Could you check a few things on this model? Use its own coordinates, in mm. A direction names the side the tool comes from. Round coordinates to 2 decimals unless told otherwise and drop trailing zeros. Write each loop counter-clockwise with the first axis right and the second up, starting at its lowest first coordinate (ties: lowest second). Pieces come first, ordered by that corner, then holes. Notation, with made-up numbers: (83.25, 73) -> (139.25, 73) arc R18 ccw to (139.25, 88) -> close; hole circle Ø6 at (36, 60.5). An arc over 180 degrees is marked (long way). Answer as CSV lines item,"result". Start each with the question number.
Q1. Imagine slicing it at C-C on y = 20. Please give me the cut outline in (x, z), and give its area (3 significant figures).
Q2. Imagine slicing it at B-B on z = 1.5. Please give me the cut outline in (x, y), and give its area (3 significant figures).
Q3. For faces 1 (the flat face through (-1, 25, 0)), 2 (the flat face through (76.5, 12, 0)), 3 (the cylindrical face through (-25.64, -0.9, 0.04)), 4 (the flat face through (76.5, -18, 0)), which set-ups out of +Z, -Z, +X, -X, +Y, -Y let a thin tool reach every point of the face, with its end or its side?
Q4. If we mould it in two halves opening along X, with no side actions, what happens to faces 5 (the flat face through (-11.5, -14, 0)), 6 (the flat face through (80, -10.5, -1)), 7 (the flat face through (-76.5, 0, 0))? For each: pulls with the +X half, pulls with the -X half, needs draft (parallel to the pull), parting line crosses it, or undercut.
Q5. If I drill on line 1 (X direction, y = -17, z = -0.1); line 2 (X direction, y = 16.5, z = 1.6); line 3 (X direction, y = -4, z = 1.8), over which ranges is the centre line in solid material (lowest first)? Write a range as [from, to].
Q6. Will this pin go through, and if not, where does the flat tip stop? pin 1 Ø1.5 at (y, z) = (-14, 0.5) entering from +X.
Q7. Imagine slicing it at A-A on y = -13.5. Please give me the cut outline in (x, z).
from build123d import *

# Parameters (mm, degrees)
SKETCH1_W           = 153
SKETCH1_H           = 50
BOSS_EXTRUDE1_DEPTH = 2.5
CUT_EXTRUDE1_DEPTH  = 6
SKETCH5_W           = 5
SKETCH5_H           = 9
BOSS_EXTRUDE2_DEPTH = 12
CUT_EXTRUDE2_DEPTH  = 9


with BuildPart() as part:
    # Sketch1 → Boss-Extrude1 (new body, symmetric)
    with BuildSketch(Plane.XY):
        Rectangle(SKETCH1_W, SKETCH1_H)
    extrude(amount=BOSS_EXTRUDE1_DEPTH, both=True)

    # Sketch2 → Cut-Extrude1 (cut, through all)
    with BuildSketch(Plane.XY.offset(2.5)):
        with BuildLine():
            Line((-26.5, -25), (-26.5, -3))
            ThreePointArc((-26.5, -3), (-25.621320344, -0.878679656), (-23.5, 0))
            Line((-23.5, 0), (-14.5, 0))
            ThreePointArc((-14.5, 0), (-12.378679656, -0.878679656), (-11.5, -3))
            Line((-11.5, -3), (-11.5, -25))
            Line((-11.5, -25), (-26.5, -25))
        make_face()
    extrude(amount=-CUT_EXTRUDE1_DEPTH, mode=Mode.SUBTRACT)

    # Sketch5 → Boss-Extrude2 (add)
    with BuildSketch(Plane(origin=(76.5, 0, 0), x_dir=(0, 0, -1), z_dir=(1, 0, 0))):
        with Locations((0, -6)):
            Rectangle(SKETCH5_W, SKETCH5_H)
    extrude(amount=BOSS_EXTRUDE2_DEPTH)

    # Sketch7 → Cut-Extrude2 (cut)
    with BuildSketch(Plane.XZ.offset(10.5)):
        Polygon((76.5, 2.5), (88.5, -2.5), (88.5, 2.5), align=None)
    extrude(amount=-CUT_EXTRUDE2_DEPTH, mode=Mode.SUBTRACT)


solid = part.part
Checks:
1,outline,"(-76.5, -2.5) -> (76.5, -2.5) -> (76.5, 2.5) -> (-76.5, 2.5) -> close"
1,area,"765 mm^2"
2,outline,"(-76.5, -25) -> (-26.5, -25) -> (-26.5, -3) arc R3 cw to (-23.5, 0) -> (-14.5, 0) arc R3 cw to (-11.5, -3) -> (-11.5, -25) -> (76.5, -25) -> (76.5, -10.5) -> (78.9, -10.5) -> (78.9, -1.5) -> (76.5, -1.5) -> (76.5, 25) -> (-76.5, 25) -> close"
2,area,"7,300 mm^2"
3,face 1,"+Z, -Z, +X, -X, +Y"
3,face 2,"+Z, -Z, +X, +Y"
3,face 3,"+Z, -Z, -Y"
3,face 4,"+Z, -Z, +X, -Y"
4,face 5,"undercut"
4,face 6,"needs draft"
4,face 7,"pulls with the -X half"
5,line 1,"[-76.5, -26.5], [-11.5, 76.5]"
5,line 2,"[-76.5, 76.5]"
5,line 3,"[-76.5, -26.5], [-11.5, 78.18]"
6,pin 1,"x = 76.5"
7,outline,"(-76.5, -2.5) -> (-26.5, -2.5) -> (-26.5, 2.5) -> (-76.5, 2.5) -> close; (-11.5, -2.5) -> (76.5, -2.5) -> (76.5, 2.5) -> (-11.5, 2.5) -> close"
